Read the model definition and answer for the solid it produces. Units are mm, in the model's axes. Face numbers are marked on the shaded views. Round coordinates to 2 decimals unless told otherwise and drop trailing zeros. Loops run counter-clockwise (first coordinate to the right, second up) from the corner with the lowest first, then second, coordinate; pieces in that order, holes last. Notation, with made-up numbers: (39, 29.5) -> (60, 29.5) arc R18 cw to (60, 57.5) -> close; hole circle Ø11 at (22.5, 47). An arc over 180 degrees is marked (long way). Put each result on its own line as item: value.
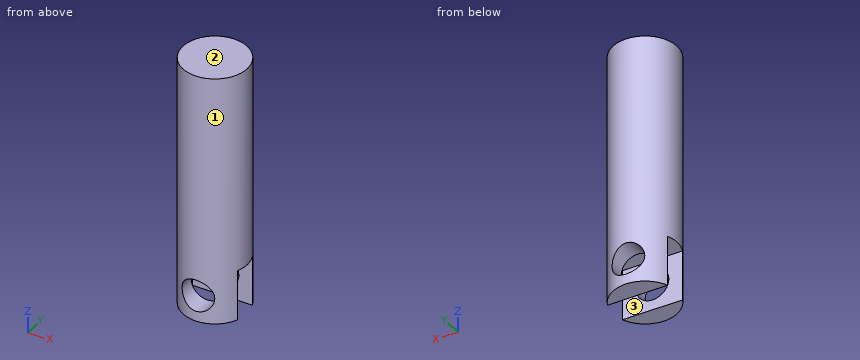
from build123d import *

# Parameters (mm, degrees)
CROQUIS1_R                 = 6.35
SALIENTE_EXTRUIR1_DEPTH    = 50
CROQUIS2_W                 = 21.76436001
CROQUIS2_H                 = 5
CORTAR_EXTRUIR1_DEPTH      = 10
CORTAR_EXTRUIR2_DEPTH      = 51.800049213
CORTAR_EXTRUIR2_DEPTH_BACK = 15.526172758
CROQUIS3_R                 = 3.175


with BuildPart() as part:
    # Croquis1 → Saliente-Extruir1 (new body)
    with BuildSketch(Plane.XY):
        Circle(CROQUIS1_R)
    extrude(amount=SALIENTE_EXTRUIR1_DEPTH)

    # Croquis2 → Cortar-Extruir1 (cut)
    with BuildSketch(Plane(origin=(0, 0, 0), x_dir=(-1, 0, 0), z_dir=(0, 0, -1))):
        Rectangle(CROQUIS2_W, CROQUIS2_H)
    extrude(amount=-CORTAR_EXTRUIR1_DEPTH, mode=Mode.SUBTRACT)

    # Croquis3 → Cortar-Extruir2 (cut, two sides: drawn at the far end of the back side and taken through both)
    with BuildSketch(Plane(origin=(0, 0, 0), x_dir=(1, 0, 0), z_dir=(0, 1, 0)).offset(-CORTAR_EXTRUIR2_DEPTH_BACK)):
        with Locations(Location((0, -5.191356095, 0), (0, 0, 270))):
            Circle(CROQUIS3_R)
    extrude(amount=CORTAR_EXTRUIR2_DEPTH + CORTAR_EXTRUIR2_DEPTH_BACK, mode=Mode.SUBTRACT)


solid = part.part
Item 1: Find the intervals of material crossed by line 1 along Z through (x, y) = (0, -3.9); line 2 along Z through (x, y) = (1, 0); line 3 along X through (y, z) = (-2.5, 29), in increasing order.
Derived:
line 1: z = 0 to 2.02, 8.37 to 50
line 2: z = 10 to 50
line 3: x = -5.84 to 5.84
Item 2: The part is cut by section A-A (x = 0). Determine the outline of the cut face in (y, z), then the cut area to 3 significant figures.
Derived:
outline: (-6.35, 0) -> (-2.5, 0) -> (-2.5, 2.02) -> (-6.35, 2.02) -> close; (-6.35, 8.37) -> (-2.5, 8.37) -> (-2.5, 10) -> (2.5, 10) -> (2.5, 8.37) -> (6.35, 8.37) -> (6.35, 50) -> (-6.35, 50) -> close; (2.5, 0) -> (6.35, 0) -> (6.35, 2.02) -> (2.5, 2.02) -> close
area: 536 mm^2
Item 3: The part is cut by section B-B (z = 4.5). Determine the outline of the cut face in (x, y).
Derived:
outline: (-5.84, -2.5) arc R6.35 ccw to (-3.1, -5.54) -> (-3.1, -2.5) -> close; (-5.84, 2.5) -> (-3.1, 2.5) -> (-3.1, 5.54) arc R6.35 ccw to start; (3.1, -5.54) arc R6.35 ccw to (5.84, -2.5) -> (3.1, -2.5) -> close; (3.1, 2.5) -> (5.84, 2.5) arc R6.35 ccw to (3.1, 5.54) -> close
Item 4: For a pull along Y with two mould halves and no side action, classify the marked faces 1, 2 and 3 as pulls with the +Y half, pulls with the -Y half, needs draft (parallel to the pull), parting line crosses it, or undercut.
Derived:
face 1: parting line crosses it
face 2: needs draft
face 3: undercut
Item 5: The part is cut by section C-C (y = -3.75). Determine the outline of the cut face in (x, z) (3 decimals), then the cut area to 3 significant figures.
Derived:
outline: (-5.124, 0) -> (5.124, 0) -> (5.124, 50) -> (-5.124, 50) -> close; hole circle Ø6.35 at (0, 5.191)
area: 481 mm^2
Item 6: Flat-ended cylindrical pins translate along their axes: pin 1 Ø3 at (y, z) = (3, 43) entering from +X; pin 2 Ø5 at (y, z) = (3.5, 17.5) entering from +X; pin 3 Ø5 at (x, z) = (1.5, 6) entering from -Y; pin 4 Ø5 at (x, z) = (0, 5.19) entering from +Y. Find the tip coordinate at first contact, or state that the pin passes through.
Derived:
pin 1: stops at x = 6.17
pin 2: stops at x = 6.27
pin 3: stops at y = -6.33
pin 4: passes through
Item 7: The part is cut by section D-D (x = -5). Determine the outline of the cut face in (y, z), then the cut area to 3 significant figures.
Derived:
outline: (-3.91, 0) -> (-2.5, 0) -> (-2.5, 10) -> (2.5, 10) -> (2.5, 0) -> (3.91, 0) -> (3.91, 50) -> (-3.91, 50) -> close
area: 341 mm^2
